```python
from build123d import *


with BuildPart() as part:
    # Skizze3 → Rotation1 (revolve)
    with BuildSketch(Plane(origin=(0, 0, 0), x_dir=(1, 0, 0), z_dir=(0, 1, 0))):
        with BuildLine():
            Line((175, 6.25), (140, 6.25))
            Line((140, 6.25), (138.75, 7.5))
            Line((138.75, 7.5), (86.859982279, 8.465395679))
            ThreePointArc((86.859982279, 8.465395679), (84.99991953, 8.491348733), (83.139695848, 8.5))
            Line((83.139695848, 8.5), (7.5, 8.5))
            Line((7.5, 8.5), (0, 8.5))
            Line((0, 8.5), (0, 0))
            Line((0, 0), (175, 0))
            Line((175, 0), (175, 6.25))
        make_face()
    revolve(axis=Axis((0, 0, 0), (-1, 0, 0)))

    # Skizze4 → Schnitt-Rotation1 (revolve, cut)
    with BuildSketch(Plane(origin=(0, 0, 0), x_dir=(1, 0, 0), z_dir=(0, 1, 0))):
        with BuildLine():
            Line((8, 8.5), (8.143933983, 8.356066017))
            ThreePointArc((8.143933983, 8.356066017), (8.25, 8.312132034), (8.356066017, 8.356066017))
            Line((8.356066017, 8.356066017), (8.5, 8.5))
            Line((8.5, 8.5), (8, 8.5))
        make_face()
    revolve(axis=Axis((0, 0, 0), (1, 0, 0)), mode=Mode.SUBTRACT)


solid = part.part
```
Read the model definition and answer for the solid it produces. Units are mm, in the model's axes. A direction names the side the tool comes from. Round coordinates to 2 decimals unless told otherwise and drop trailing zeros. Write each loop counter-clockwise with the first axis right and the second up, starting at its lowest first coordinate (ties: lowest second). Pieces come first, ordered by that corner, then holes. Notation, with made-up numbers: (26.5, 54.25) -> (33.5, 54.25) arc R8 ccw to (33.5, 59.25) -> close; hole circle Ø2 at (84.25, 44). An arc over 180 degrees is marked (long way). Answer in a Markdown table with one row per item. Add a question column.
1) Find section A-A, the plane x = 151.5. Determine the outline of the cut face in (y, z), and give its area (3 significant figures).
2) Find section B-B, the plane x = 124. Determine the outline of the cut face in (y, z).
3) Consider line 1 (Z direction, x = 151, y = 0.5); line 2 (Z direction, x = 42.5, y = 0.25); line 3 (Y direction, x = 55, z = 3.75). Determine where each line is inside the solid, lowest interval first.
4) Given P1, Ø6, axis at x = 147, z = -0.5, coming from the -Y side; P2, Ø3, axis at y = -6.5, z = 6, coming from the +X side; P3, Ø6, axis at x = 59, z = 5, coming from the +Y side, each flat-ended and moving along its own axis, determine where each tip first touches the part or whether it passes through.
5) Which of the six approach directions +Z, -Z, +X, -X, +Y, -Y give full straight-line access (tool end or side, diameter ignored) to faces 1 (the face through (112.44, 7.8, 1.73)), 2 (the face through (3.944, -7.167, -4.57))?
Findings below:
| question | item | result |
|---|---|---|
| 1 | outline | circle Ø12.5 at (0, 0) |
| 1 | area | 123 mm² |
| 2 | outline | circle Ø15.55 at (0, 0) |
| 3 | line 1 | -6.23 to 6.23 |
| 3 | line 2 | -8.5 to 8.5 |
| 3 | line 3 | -7.63 to 7.63 |
| 4 | P1 | y = -6.25 |
| 4 | P2 | x = 138.9 |
| 4 | P3 | y = 8.26 |
| 5 | face 1 | +X |
| 5 | face 2 | +X, -X |
